Check sheet for the modelled part. Datum: model origin and axes. Units: mm. Face numbers are marked on the shaded views. Round coordinates to 2 decimals unless told otherwise and drop trailing zeros. Order: outer loops, then holes, each group sorted by start corner. A loop starts at its lowest first (then second) coordinate and runs counter-clockwise, first axis right, second up.
```python
from build123d import *

# Parameters (mm, degrees)
F2_R     = 16.5358805208
F2_R_2   = 8.5
F3_DEPTH = 1
F4_R     = 15.1866700875
F4_R_2   = 11.3
F5_DEPTH = 2
F6_R     = 1.99999


# Not quite as in the source:
# - a fillet or chamfer is up to 0.001 mm smaller than in the source, because OpenCascade refuses the exact size


with BuildPart() as f1:
    # F0 (on Front) → F1 (revolve)
    with BuildSketch(Plane.XZ):
        with BuildLine():
            ThreePointArc((13.5358805208, -4), (12.3077325791, -0.0459885139), (13.1866700875, 4))
            Line((13.1866700875, 4), (11.3, 4))
            Line((11.3, 4), (11.3, -4))
            Line((11.3, -4), (13.5358805208, -4))
        make_face()
    revolve(axis=Axis((0, 0, -1.1675134301), (0, 0, -1)))

    # F2 (on face) → F3 (join)
    with BuildSketch(Plane(origin=(0, 0, -4), x_dir=(1, 0, 0), z_dir=(0, 0, -1))):
        Circle(F2_R)
        Circle(F2_R_2, mode=Mode.SUBTRACT)
    extrude(amount=F3_DEPTH)

    # F4 (on face) → F5 (join)
    with BuildSketch(Plane.XY.offset(4)):
        Circle(F4_R)
        Circle(F4_R_2, mode=Mode.SUBTRACT)
    extrude(amount=F5_DEPTH)

    # F6 (radius 2 in the source; OpenCascade refuses exactly that, so slightly less here)
    f6_edges = [f1.edges().sort_by_distance(p)[0] for p in [
        (-15.18667, 0, 4),
    ]]
    fillet(f6_edges, radius=F6_R)


solid = f1.part
```
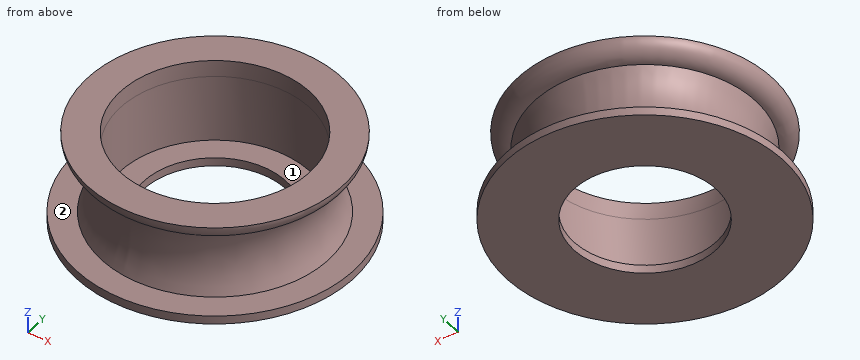
Item 1: Scan lines: line 1 along X through (y, z) = (0, -4.4); line 2 along X through (y, z) = (0, -1.75). Record each from-to range of solid material in increasing order.
Answer:
line 1: x = -16.54 to -8.5, 8.5 to 16.54
line 2: x = -12.56 to -11.3, 11.3 to 12.56
Item 2: Sectioned sample at D-D (z = -0.25). Record the cut outline in (x, y), and give its area (3 significant figures).
Answer:
outline: circle Ø24.64 at (0, 0); hole circle Ø22.6 at (0, 0)
area: 75.6 mm2
Item 3: Go/stop test with flat-tipped pins: P1, Ø4, axis at x = 3.5, z = 3, coming from the +Y side; P2, Ø6, axis at y = 4, z = -0.5, coming from the +X side; P3, Ø3, axis at x = 3, z = 4, coming from the +Y side. Record where each tip stops, or that it passes through.
Answer:
P1: stops at y = 14.58
P2: stops at x = 12.82
P3: stops at y = 14.89
Item 4: Sectioned sample at C-C (z = 4.5). Record the cut outline in (x, y), and give its area (3 significant figures).
Answer:
outline: circle Ø29.02 at (0, 0); hole circle Ø22.6 at (0, 0)
area: 260 mm2
Item 5: Release check for a two-part mould opening along X. For the marked faces 1 and 2 record: released by +X, released by -X, zero draft, split by the parting line, or undercut.
Answer:
face 1: undercut
face 2: zero draft
